The listing builds one solid part. Answer for the finished solid, in the listing's coordinates (mm). Face numbers are marked on the shaded views. A direction names the side the tool comes from. Coordinates: 2 decimals unless noted, no trailing zeros. Loops run counter-clockwise (first coordinate to the right, second up) from the corner with the lowest first, then second, coordinate; pieces in that order, holes last. Notation, with made-up numbers: (-9.5, 79.5) - (-0.5, 79.5) arc R30 cw to (-0.5, 104.5) - close; hole circle Ø6 at (56, -27). An arc over 180 degrees is marked (long way). Write each question's results on one line, items separated by ' | '. Start each with the question number.
(1) Find section D-D on y = 32. State how many separate pieces and enclosed holes the cut face has, then the cut area to 3 significant figures.
(2) Given pin 1 Ø6 at (x, y) = (-124.5, 10) entering from -Z; pin 2 Ø3.5 at (y, z) = (35.5, -67.5) entering from +X; pin 3 Ø0.8 at (y, z) = (51, -68.5) entering from +X; pin 4 Ø12 at (x, z) = (-137.5, -47.5) entering from +Y, each flat-ended and moving along its own axis, determine where each tip first touches the part or whether it passes through.
(3) For the marked faces 1, 2 and 3, determine the directions among +Z, -Z, +X, -X, +Y, -Y from which every point of the face is accessible in a straight line to the end or side of a thin tool.
(4) Consider line 1 (Z direction, x = -123.5, y = 25.5); line 2 (X direction, y = 44.5, z = -75.5); line 3 (Y direction, x = -164.5, z = -49). Determine where each line is inside the solid, lowest interval first. Write a range as from..to.
(5) Find section A-A on z = -79. Determine the outline of the cut face in (x, y).
(6) Find section C-C on z = -45.5. Determine the outline of the cut face in (x, y).
(7) Find section B-B on x = -152. Determine the outline of the cut face in (y, z), then the cut area to 3 significant figures.
Autodesk Inventor part; units mm, degrees
ref_plane "YZ Plane" through (0, 0, 0) normal (1, 0, 0) x (0, 1, 0)
ref_plane "XZ Plane" through (0, 0, 0) normal (0, 1, 0) x (-1, 0, 0)
ref_plane "XY Plane" through (0, 0, 0) normal (0, 0, 1) x (1, 0, 0)
sketch "Sketch1" plane through (0, 0, 0) normal (0, 1, 0) x (-1, 0, 0)
  circle A0 centre (145.0721, -68.2626) radius 28.4988
  arc A1 (147.6629, -66.2154) -> (147.6629, -70.3098) centre (145.0721, -68.2626) ccw
  line L0 (147.6629, -70.3098) -> (147.6629, -66.2154)
  circle A2 centre (144.9959, -92.0115) radius 2.794
  circle A3 centre (145.1103, -44.4477) radius 2.794
  circle A4 centre (165.6011, -80.2031) radius 2.794
  circle A5 centre (124.4669, -56.3221) radius 2.794
  circle A6 centre (165.6773, -56.4542) radius 2.794
  circle A7 centre (124.4287, -80.137) radius 2.794
  circle A8 centre (145.1483, -44.5137) radius 2.794
  circle A9 centre (145.0339, -92.0776) radius 2.794
  circle A10 centre (124.5431, -56.3222) radius 2.794
  circle A11 centre (165.6773, -80.2032) radius 2.794
  circle A12 centre (124.4669, -80.0711) radius 2.794
  circle A13 centre (165.7155, -56.3882) radius 2.794
  circle A14 centre (151.9123, -75.1789) radius 1.9685
  circle A15 centre (151.9884, -61.4224) radius 1.9685
  circle A16 centre (138.2319, -61.3463) radius 1.9685
  circle A17 centre (138.1558, -75.1028) radius 1.9685
  point P0 (0, 0)
  dimension "d1" = 6.604
  dimension "d3" = 5.588
  dimension "d4" = 23.749
  dimension "d7" = 360
  dimension "d9" = 3.937
  dimension "d14" = 360
  dimension "d25" = 2.5908
extrude "Extrusion1" add sketch "Sketch1" along normal blind 50.038 contours A0 | A2 A9 | A3 A8 | A4 A11 | A5 A10 | A6 A13 | A7 A12 picked at (146.4388, -94.4143) picked at (146.5538, -46.8501) picked at (168.4221, -80.4123) picked at (127.2879, -56.5313) picked at (167.123, -54.0531) picked at (125.875, -77.7363)
sketch "Sketch2" plane through (-145.0721, 50.038, -68.2626) normal (0, 1, 0) x (1, 0, 0)
  circle A0 centre (0, 0) radius 11.8872
  circle A1 centre (0, 0) radius 28.4988
  point P0 (145.0721, -68.2626)
  dimension "d18" = 23.7744
extrude "Extrusion2" cut sketch "Sketch2" against normal blind 2.032
sketch "Sketch3" plane through (-145.0721, 0, -68.2626) normal (0, -1, 0) x (1, 0, 0)
  arc A0 (-2.5908, -2.0472) -> (-2.5908, 2.0472) centre (0, 0) ccw
  circle A1 centre (0, 0) radius 11.8872
  circle A2 centre (0, 0) radius 28.4988
  point P0 (145.0721, 68.2626)
extrude "Extrusion3" cut sketch "Sketch3" against normal blind 2.032
sketch "Sketch4" plane through (-145.0721, 50.038, -68.2626) normal (0, 1, 0) x (1, 0, 0)
  circle A0 centre (0, 0) radius 11.8872 construction
  circle A1 centre (6.9163, 6.8402) radius 1.9685 construction
  circle A2 centre (-6.8402, 6.9163) radius 1.9685 construction
  circle A3 centre (-6.9163, -6.8402) radius 1.9685 construction
  circle A4 centre (6.8402, -6.9163) radius 1.9685 construction
  arc A5 (-2.5908, -2.0472) -> (-2.5908, 2.0472) centre (0, 0) ccw construction
  line L0 (-2.5908, -2.0472) -> (-2.5908, 2.0472) construction
  arc A6 (-2.5908, -2.0472) -> (-2.5908, 2.0472) centre (0, 0) ccw
  arc A7 (-2.5908, -2.0472) -> (-2.5908, 2.0472) centre (0, 0) ccw
  circle A8 centre (0, 0) radius 11.8872
  circle A9 centre (-6.8402, 6.9163) radius 1.9685
  circle A10 centre (6.9163, 6.8402) radius 1.9685
  circle A11 centre (6.9163, 6.8402) radius 1.9685
  circle A12 centre (-6.9163, -6.8402) radius 1.9685
  circle A13 centre (6.8402, -6.9163) radius 1.9685
  line L1 (-2.5908, 2.0472) -> (-2.5908, -2.0472)
  point P0 (145.0721, -68.2626)
  dimension "d26" = 3.302
  dimension "d27" = 2.5908
extrude "Extrusion4" add sketch "Sketch4" along normal blind 2.54
properties part number "wheel insert"
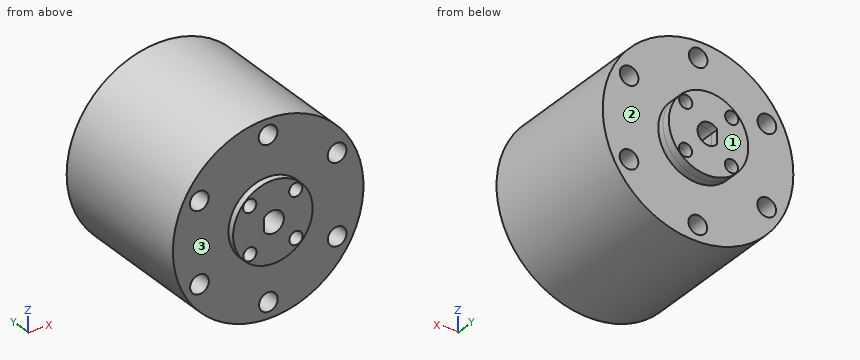
Values:
1) separate pieces: 1 | enclosed holes: 11 | area: 2,320 mm²
2) pin 1: stops at z = -90.7 | pin 2: stops at x = -116.57 | pin 3: stops at x = -133.18 | pin 4: stops at y = 48.01
3) face 1: +Z, -Z, +X, -X, +Y | face 2: +Y | face 3: -Y
4) line 1: z = -86.89..-82.77, -77.5..-58.94, -53.7..-49.64 | line 2: x = -172.64..-153.85, -149.97..-140.08, -136.23..-117.51 | line 3: y = 2.03..48.01
5) outline: (-171.47, 2.03) - (-168.12, 2.03) - (-168.12, 48.01) - (-171.47, 48.01) - close; (-163.08, 2.03) - (-150.17, 2.03) - (-150.17, 0) - (-139.97, 0) - (-139.97, 2.03) - (-126.98, 2.03) - (-126.98, 48.01) - (-139.97, 48.01) - (-139.97, 52.58) - (-150.17, 52.58) - (-150.17, 48.01) - (-163.08, 48.01) - close; (-121.88, 2.03) - (-118.67, 2.03) - (-118.67, 48.01) - (-121.88, 48.01) - close
6) outline: (-162.22, 2.03) - (-147.7, 2.03) - (-147.7, 48.01) - (-162.22, 48.01) - close; (-142.52, 2.03) - (-127.92, 2.03) - (-127.92, 48.01) - (-142.52, 48.01) - close
7) outline: (0, -77.92) - (2.03, -77.92) - (2.03, -95.91) - (48.01, -95.91) - (48.01, -77.92) - (52.58, -77.92) - (52.58, -77.15) - (0, -77.15) - close; (0, -73.21) - (52.58, -73.21) - (52.58, -63.39) - (0, -63.39) - close; (0, -59.45) - (52.58, -59.45) - (52.58, -58.6) - (48.01, -58.6) - (48.01, -40.62) - (2.03, -40.62) - (2.03, -58.6) - (0, -58.6) - close | area: 2,260 mm²
